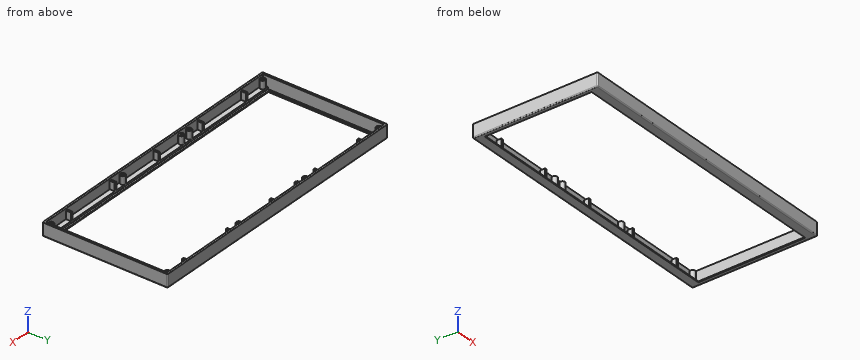
from build123d import *

# Parameters (mm, degrees)
SKETCH012_W     = 281.5
SKETCH012_H     = 125
PAD006_DEPTH    = 13
SKETCH013_W     = 277.5
SKETCH013_H     = 111
POCKET003_DEPTH = 12
SKETCH014_W     = 273.5
SKETCH014_H     = 107
POCKET004_DEPTH = 1.001
SKETCH015_W     = 277.5
SKETCH015_H     = 121
POCKET005_DEPTH = 10
SKETCH016_R     = 2.5
SKETCH016_W     = 2
SKETCH016_H     = 5
PAD_DEPTH       = 8
SKETCH_R        = 0.9
POCKET_DEPTH    = 8
FILLET_R        = 1


with BuildPart() as part:
    # Sketch012 → Pad006 (new body)
    with BuildSketch(Plane.XY):
        Rectangle(SKETCH012_W, SKETCH012_H)
    extrude(amount=PAD006_DEPTH)

    # Sketch013 (on Face6 of Pad006) → Pocket003 (cut)
    with BuildSketch(Plane.XY.offset(13)):
        Rectangle(SKETCH013_W, SKETCH013_H)
    extrude(amount=-POCKET003_DEPTH, mode=Mode.SUBTRACT)

    # Sketch014 (on Face11 of Pocket003) → Pocket004 (cut, through all)
    with BuildSketch(Plane.XY.offset(1)):
        Rectangle(SKETCH014_W, SKETCH014_H)
    extrude(amount=-POCKET004_DEPTH, mode=Mode.SUBTRACT)

    # Sketch015 (on Face5 of Pocket004) → Pocket005 (cut)
    with BuildSketch(Plane.XY.offset(13)):
        Rectangle(SKETCH015_W, SKETCH015_H)
    extrude(amount=-POCKET005_DEPTH, mode=Mode.SUBTRACT)

    # Sketch016 (on Face14 of Pocket005) → Pad (join)
    with BuildSketch(Plane.XY.offset(3)):
        with Locations((-135.25, 58)):
            Circle(SKETCH016_R)
        with Locations((-135.25, -58)):
            Circle(SKETCH016_R)
        with Locations((-41.25, 58)):
            Circle(SKETCH016_R)
        with Locations((43.75, 58)):
            Circle(SKETCH016_R)
        with Locations((-41.25, -58)):
            Circle(SKETCH016_R)
        with Locations((43.75, -58)):
            Circle(SKETCH016_R)
        with Locations((135.25, 58)):
            Circle(SKETCH016_R)
        with Locations((135.25, -58)):
            Circle(SKETCH016_R)
        with Locations((-31.25, 58)):
            Circle(SKETCH016_R)
        with Locations((-31.25, -58)):
            Circle(SKETCH016_R)
        with Locations((-111.75, 58)):
            Rectangle(SKETCH016_W, SKETCH016_H)
        with Locations((-55.75, 58)):
            Rectangle(SKETCH016_W, SKETCH016_H)
        with Locations((0.25, 58)):
            Rectangle(SKETCH016_W, SKETCH016_H)
        with Locations((56.25, 58)):
            Rectangle(SKETCH016_W, SKETCH016_H)
        with Locations((112.25, 58)):
            Rectangle(SKETCH016_W, SKETCH016_H)
        with Locations((-111.75, -58)):
            Rectangle(SKETCH016_W, SKETCH016_H)
        with Locations((-55.75, -58)):
            Rectangle(SKETCH016_W, SKETCH016_H)
        with Locations((0.25, -58)):
            Rectangle(SKETCH016_W, SKETCH016_H)
        with Locations((56.25, -58)):
            Rectangle(SKETCH016_W, SKETCH016_H)
        with Locations((112.25, -58)):
            Rectangle(SKETCH016_W, SKETCH016_H)
    extrude(amount=PAD_DEPTH)

    # Sketch (on Face9 of Pad) → Pocket (cut)
    with BuildSketch(Plane.XY.offset(11)):
        with Locations((-135.25, 58)):
            Circle(SKETCH_R)
        with Locations((-41.25, 58)):
            Circle(SKETCH_R)
        with Locations((-31.25, 58)):
            Circle(SKETCH_R)
        with Locations((43.75, 58)):
            Circle(SKETCH_R)
        with Locations((135.25, 58)):
            Circle(SKETCH_R)
        with Locations((135.25, -58)):
            Circle(SKETCH_R)
        with Locations((43.75, -58)):
            Circle(SKETCH_R)
        with Locations((-31.25, -58)):
            Circle(SKETCH_R)
        with Locations((-41.25, -58)):
            Circle(SKETCH_R)
        with Locations((-135.25, -58)):
            Circle(SKETCH_R)
    extrude(amount=-POCKET_DEPTH, mode=Mode.SUBTRACT)

    # Fillet
    fillet_edges = [part.edges().sort_by_distance(p)[0] for p in [
        (-140.75, 0, 0),
        (-140.75, 62.5, 6.5),
        (0, 62.5, 0),
        (-140.75, -62.5, 6.5),
        (0, -62.5, 0),
        (140.75, -62.5, 6.5),
        (140.75, 0, 0),
        (140.75, 62.5, 6.5),
    ]]
    fillet(fillet_edges, radius=FILLET_R)


solid = part.part
Work out the finished part from the listing and answer in its coordinate system (mm). Give positions to 0.01 mm unless a question says otherwise; leave off trailing zeros. Write each loop counter-clockwise with the first axis right and the second up, starting at its lowest first coordinate (ties: lowest second). Pieces come first, ordered by that corner, then holes.
Q1. The part is cut by section A-A on x = 67. Give the vertices of the cut face in (y, z).
Answer:
outline: (-62.5, 1) arc R1 ccw to (-61.5, 0) - (-53.5, 0) - (-53.5, 1) - (-55.5, 1) - (-55.5, 3) - (-60.5, 3) - (-60.5, 13) - (-62.5, 13) - close; (53.5, 0) - (61.5, 0) arc R1 ccw to (62.5, 1) - (62.5, 13) - (60.5, 13) - (60.5, 3) - (55.5, 3) - (55.5, 1) - (53.5, 1) - close
Q2. The part is cut by section B-B on y = 49.5. Give the vertices of the cut face in (x, z), and give its area (3 significant figures).
Answer:
outline: (-140.75, 1) arc R1 ccw to (-139.75, 0) - (-136.75, 0) - (-136.75, 1) - (-138.75, 1) - (-138.75, 13) - (-140.75, 13) - close; (136.75, 0) - (139.75, 0) arc R1 ccw to (140.75, 1) - (140.75, 13) - (138.75, 13) - (138.75, 1) - (136.75, 1) - close
area: 55.6 mm2
Q3. Straight lines are drawn through the part: L1, parallel to X at y = -43, z = 6.75; L2, parallel to Y at x = -89.5, z = 7; L3, parallel to Y at x = -19.5, z = 1.25. For each, find the intervals that lie inside material, in ascending order.
Answer:
L1: x = -140.75 to -138.75, 138.75 to 140.75
L2: y = -62.5 to -60.5, 60.5 to 62.5
L3: y = -62.5 to -55.5, 55.5 to 62.5
Q4. Given pin 1 (5.5 mm diameter, centred on x = -32, y = -57.5, fed in from +Z); pin 2 (0.5 mm diameter, centred on x = 27, z = 0.5, fed in from -Y); pin 3 (5.5 mm diameter, centred on x = 92.5, y = 59, fed in from +Z), each flat-ended and moving along its own axis, determine where each tip first touches the part or whether it passes through.
Answer:
pin 1: stops at z = 11
pin 2: stops at y = -62.47
pin 3: stops at z = 13
